from build123d import *

# Parameters (mm, degrees)
SKETCH1_R                      = 72.5
BOSS_EXTRUDE1_DEPTH            = 42
SKETCH2_R                      = 48.2
BOSS_EXTRUDE2_DEPTH            = 33
SKETCH4_R                      = 28.6
CUT_EXTRUDE1_DEPTH             = 156.568312969
SKETCH5_R                      = 35
CUT_EXTRUDE2_DEPTH             = 8
SKETCH6_W                      = 12.5
SKETCH6_H                      = 6
FILLET1_R                      = 5
SKETCH7_R                      = 5.35
CUT_EXTRUDE3_DEPTH             = 156.568312969
CIRPATTERN1_COUNT              = 12
CHAMFER1_SIZE                  = 2
CUT_EXTRUDE4_DEPTH             = 177.599830124
CUT_EXTRUDE4_DEPTH_BACK        = 1.6
SKETCH8_W                      = 51
SKETCH8_H                      = 63
BOSS_EXTRUDE3_START            = -42
SKETCH10_R                     = 5.35
BOSS_EXTRUDE3_DEPTH            = 42
SKETCH9_R                      = 19
CUT_EXTRUDE5_DEPTH             = 1.6
SKETCH11_R                     = 12.4
CUT_EXTRUDE6_DEPTH             = 23
CUT_EXTRUDE7_REACH             = 158.227
CUT_EXTRUDE7_END_RADIUS        = 28.6
SKETCH12_R                     = 7.5
CUT_EXTRUDE7_DIRECTION_2_DEPTH = 157.227206337
CUT_EXTRUDE8_REACH             = 157.568
CUT_EXTRUDE8_END_RADIUS        = 7.5
SKETCH13_R                     = 3
CHAMFER2_SIZE                  = 1
CUT_EXTRUDE11_START            = 41.236068177
CUT_EXTRUDE11_DEPTH            = 6.963931924


# Read off the part's stored shape, not the designer's step: Cut-Extrude11
with BuildPart() as part:
    # Sketch1 → Boss-Extrude1 (new body)
    with BuildSketch(Plane.XY):
        with Locations(Location((0, 0, 0), (0, 0, 180))):
            Circle(SKETCH1_R)
    extrude(amount=BOSS_EXTRUDE1_DEPTH)

    # Sketch2 → Boss-Extrude2 (add)
    with BuildSketch(Plane.XY.offset(42)):
        Circle(SKETCH2_R)
    extrude(amount=BOSS_EXTRUDE2_DEPTH)

    # Sketch3 → Revolve1 (revolve)
    with BuildSketch(Plane(origin=(0, 0, 0), x_dir=(0, 0, -1), z_dir=(1, 0, 0)), mode=Mode.PRIVATE) as revolve1_sk:
        Polygon((0, 47.6), (42, 41.5), (42, 28.6), (0, 28.6), align=None)
    revolve(revolve1_sk.sketch.rotate(Axis((0, 0, 0), (0, 0, -1)), 90), axis=Axis((0, 0, 0), (0, 0, -1)))

    # Sketch4 → Cut-Extrude1 (cut, through all)
    with BuildSketch(Plane.XY.offset(75)):
        Circle(SKETCH4_R)
    extrude(amount=-CUT_EXTRUDE1_DEPTH, mode=Mode.SUBTRACT)

    # Sketch5 → Cut-Extrude2 (cut)
    with BuildSketch(Plane(origin=(0, 0, -42), x_dir=(-1, 0, 0), z_dir=(0, 0, -1))):
        Circle(SKETCH5_R)
    extrude(amount=-CUT_EXTRUDE2_DEPTH, mode=Mode.SUBTRACT)

    # Sketch6 → Cut-Revolve1 (revolve, cut)
    with BuildSketch(Plane(origin=(0, 0, 0), x_dir=(0, 0, -1), z_dir=(1, 0, 0)), mode=Mode.PRIVATE) as cut_revolve1_sk:
        with Locations((-58.75, 45.2)):
            Rectangle(SKETCH6_W, SKETCH6_H)
    revolve(cut_revolve1_sk.sketch.rotate(Axis((0, 0, 75), (0, 0, -1)), 90), axis=Axis((0, 0, 75), (0, 0, -1)), mode=Mode.SUBTRACT)

    # Fillet1
    fillet1_edges = [part.edges().sort_by_distance(p)[0] for p in [
        (-41.5, 0, -42),
    ]]
    fillet(fillet1_edges, radius=FILLET1_R)

    # Sketch7 → Cut-Extrude3 (cut, through all)
    with BuildSketch(Plane.XY.offset(75)):
        with Locations((0, 62.5)):
            Circle(SKETCH7_R)
    cut_extrude3 = extrude(amount=-CUT_EXTRUDE3_DEPTH, mode=Mode.SUBTRACT)

    # CirPattern1: Cut-Extrude3 ×12 about axis
    cirpattern1_axis = Axis((0, 0, 0), (0, 0, 1))
    for i in range(1, CIRPATTERN1_COUNT):
        add(cut_extrude3.rotate(cirpattern1_axis, i * 360 / CIRPATTERN1_COUNT), mode=Mode.SUBTRACT)

    # Chamfer1
    chamfer1_edges = [part.edges().sort_by_distance(p)[0] for p in [
        (-28.6, 0, 75),
    ]]
    chamfer(chamfer1_edges, length=CHAMFER1_SIZE)

    # Sketch8 → Cut-Extrude4 (cut, two sides: drawn at the far end of the back side and taken through both)
    with BuildSketch(Plane(origin=(0, 70, 0), x_dir=(1, 0, 0), z_dir=(0, 1, 0)).offset(-CUT_EXTRUDE4_DEPTH_BACK)):
        with Locations((0, -21)):
            Rectangle(SKETCH8_W, SKETCH8_H)
    extrude(amount=CUT_EXTRUDE4_DEPTH + CUT_EXTRUDE4_DEPTH_BACK, mode=Mode.SUBTRACT)

    # Sketch10 → Boss-Extrude3 (add)
    with BuildSketch(Plane(origin=(0, 0, 0), x_dir=(-1, 0, 0), z_dir=(0, 0, -1)).offset(BOSS_EXTRUDE3_START)):
        with Locations((0, 62.5)):
            Circle(SKETCH10_R)
    extrude(amount=BOSS_EXTRUDE3_DEPTH)

    # Sketch9 → Cut-Extrude5 (cut)
    with BuildSketch(Plane(origin=(0, 68.4, 0), x_dir=(1, 0, 0), z_dir=(0, 1, 0))):
        with Locations(Location((0, -21, 0), (0, 0, 270))):
            Circle(SKETCH9_R)
    extrude(amount=-CUT_EXTRUDE5_DEPTH, mode=Mode.SUBTRACT)

    # Sketch11 → Cut-Extrude6 (cut)
    with BuildSketch(Plane(origin=(0, 66.8, 0), x_dir=(1, 0, 0), z_dir=(0, 1, 0))):
        with Locations(Location((0, -21, 0), (0, 0, 270))):
            Circle(SKETCH11_R)
    extrude(amount=-CUT_EXTRUDE6_DEPTH, mode=Mode.SUBTRACT)

    # Cut-Extrude7: up to this cylinder (the profile starts outside it)
    cut_extrude7_end = Plane(origin=(0, 0, 21), z_dir=(0, 0, 1)) * Cylinder(CUT_EXTRUDE7_END_RADIUS, 374.654, mode=Mode.PRIVATE)
    # Sketch12 → Cut-Extrude7 (cut, up to the surface)
    with BuildSketch(Plane(origin=(0, 43.8, 0), x_dir=(1, 0, 0), z_dir=(0, 1, 0)), mode=Mode.PRIVATE) as cut_extrude7_sk1:
        with Locations(Location((0, -21, 0), (0, 0, 270))):
            Circle(SKETCH12_R)
    cut_extrude7_tool1 = extrude(cut_extrude7_sk1.sketch, amount=-CUT_EXTRUDE7_REACH, mode=Mode.PRIVATE) - cut_extrude7_end
    add(cut_extrude7_tool1.solids().sort_by_distance((0, 43.8, 21))[0], mode=Mode.SUBTRACT)

    # Sketch12 → Cut-Extrude7 direction 2 (cut)
    with BuildSketch(Plane(origin=(0, 43.8, 0), x_dir=(1, 0, 0), z_dir=(0, 1, 0))):
        with Locations(Location((0, -21, 0), (0, 0, 270))):
            Circle(SKETCH12_R)
    extrude(amount=CUT_EXTRUDE7_DIRECTION_2_DEPTH, mode=Mode.SUBTRACT)

    # Cut-Extrude8: up to this cylinder (the profile starts outside it)
    cut_extrude8_end = Plane(origin=(0, 39, 21), z_dir=(0, -1, 0)) * Cylinder(CUT_EXTRUDE8_END_RADIUS, 331.136, mode=Mode.PRIVATE)
    # Sketch13 → Cut-Extrude8 (cut, up to the surface)
    with BuildSketch(Plane.XY.offset(75), mode=Mode.PRIVATE) as cut_extrude8_sk1:
        with Locations((0, 39)):
            Circle(SKETCH13_R)
    cut_extrude8_tool1 = extrude(cut_extrude8_sk1.sketch, amount=-CUT_EXTRUDE8_REACH, mode=Mode.PRIVATE) - cut_extrude8_end
    add(cut_extrude8_tool1.solids().sort_by_distance((0, 39, 75))[0], mode=Mode.SUBTRACT)

    # Chamfer2
    chamfer2_edges = [part.edges().sort_by_distance(p)[0] for p in [
        (-3, 39, 75),
    ]]
    chamfer(chamfer2_edges, length=CHAMFER2_SIZE)

    # Cut-Extrude11 outline → Cut-Extrude11 (cut)
    with BuildSketch(Plane(origin=(0, 0, 0), x_dir=(1, 0, 0), z_dir=(0, 1, 0)).offset(CUT_EXTRUDE11_START)):
        with BuildLine():
            add(Edge.make_bspline(
                [(0, -68), (-0.54702537, -68), (-1.060578619, -68.230628831), (-1.773892363, -68.947000843), (-1.998941239, -69.453645947), (-2.001051196, -70.538574914), (-1.778362753, -71.046998742), (-1.061992496, -71.769449741), (-0.543253329, -71.998843249), (0.534702492, -72.001147611), (1.060100727, -71.770006855), (1.774982575, -71.051748391), (1.999780329, -70.547535826), (2.000219348, -69.454070146), (1.774866101, -68.94836038), (1.061104675, -68.230776319), (0.54702537, -68), (0, -68)],
                knots=[0, 0, 0, 0, 0.125, 0.125, 0.25, 0.25, 0.375, 0.375, 0.5, 0.5, 0.625, 0.625, 0.75, 0.75, 0.875, 0.875, 1, 1, 1, 1], degree=3))
        make_face()
    extrude(amount=CUT_EXTRUDE11_DEPTH, mode=Mode.SUBTRACT)


solid = part.part
Source: CAD feature listing. Evaluate the final solid. Frame: model axes, mm. A direction names the side the tool comes from. Round coordinates to 2 decimals unless told otherwise and drop trailing zeros. Order: outer loops, then holes, each group sorted by start corner. A loop starts at its lowest first (then second) coordinate and runs counter-clockwise, first axis right, second up. Notation, with made-up numbers: (-34.75, -14.5) - (20.25, -14.5) arc R30 ccw to (20.25, 19.5) - close; hole circle Ø7 at (20.5, -25). An arc over 180 degrees is marked (long way). Use a Markdown table: item, result. Add a question column.
1. First-contact query: pin 1 (8.5 mm diameter, centred on x = -31.25, y = 54.13, fed in from +Z); pin 2 (14 mm diameter, centred on x = 31.25, y = 54.13, fed in from -Z); pin 3 (14 mm diameter, centred on x = 62.5, y = 0, fed in from +Z); pin 4 (1 mm diameter, centred on x = 54, z = 14, fed in from -Y). Flat tips, straight axial feed; report the tip coordinate or a pass-through.
2. Mould query, pull axis X, two halves, no side actions, for faces 1 (the cylindrical face through (57.003, -26.739, 21.294)), 2 (the flat face through (-12, 66.8, 25)), 3 (the flat face through (-15, 46, 42)). Classes: +X half, -X half, draft (parallel to the pull), parting line (faces both ways), or undercut.
3. Set-up query: faces 4 (the cylindrical face through (67.804, 0.696, 21.294)), 5 (the cylindrical face through (1.384, 36.338, 51.26)), 6 (the flat face through (33.24, -34.35, 0)), 7 (the cylindrical face through (0.33, 35.813, 13.507)), 8 (the flat face through (0, 43, 52.5)). Return all of +Z, -Z, +X, -X, +Y, -Y with unobstructed straight access to the full face (end or side cutting, diameter ignored); none if empty.
4. Section query C-C (y = 0). Give the number of separate pieces and of enclosed holes in the cut face, then the cut area to 3 significant figures.
5. Line query: probe 1 along Y at (x, z) = (-30.5, 37); probe 2 along X at (y, z) = (-35, 38); probe 3 along Y at (x, z) = (0, 19). Output: solid intervals per line, ascending.
6. Section query A-A (x = 62.5). Return the cut outline in (y, z), then the cut area to 3 significant figures.
Derived:
| question | item | result |
|---|---|---|
| 1 | pin 1 | through |
| 1 | pin 2 | z = 0 |
| 1 | pin 3 | z = 42 |
| 1 | pin 4 | y = -48.93 |
| 2 | face 1 | undercut |
| 2 | face 2 | undercut |
| 2 | face 3 | draft |
| 3 | face 4 | +Z, -Z |
| 3 | face 5 | +Z |
| 3 | face 6 | -Z |
| 3 | face 7 | +Y |
| 3 | face 8 | none |
| 4 | separate pieces | 4 |
| 4 | enclosed holes | 0 |
| 4 | area | 5,160 mm2 |
| 5 | probe 1 | -65.77 to -59.42, -48.83 to 48.83, 59.42 to 65.77 |
| 5 | probe 2 | -63.49 to -57.94, -50.31 to 50.31, 57.94 to 63.49 |
| 5 | probe 3 | -72.5 to -67.85, -57.15 to -28.6 |
| 6 | outline | (-36.74, 0) - (-5.35, 0) - (-5.35, 42) - (-36.74, 42) - close; (5.35, 0) - (36.74, 0) - (36.74, 42) - (5.35, 42) - close |
| 6 | area | 2,640 mm2 |
